from build123d import *

# Parameters (mm, degrees)
F0_R      = 5.1
F1_DEPTH  = 35
F3_START  = -5
F2_W      = 22
F2_H      = 9.65
F3_DEPTH  = 30
F4_DEPTH  = 2.5
F5_R      = 1.9
F6_DEPTH  = 20
F5_R_2    = 2.65
F7_DEPTH  = 2
F9_DEPTH  = 35
F10_COUNT = 3
F10_ANGLE = 240


with BuildPart() as f1:
    # F0 (on Top) → F1 (new body)
    with BuildSketch(Plane.XY):
        with BuildLine():
            Line((48.3891499996, -27.9374887781), (0, 0))
            Line((0, 0), (-48.3891499996, -27.9374887781))
            ThreePointArc((-48.3891499996, -27.9374887781), (-37.0005953155, -59.5433683199), (-37.3249107961, -93.1369036932))
            ThreePointArc((-37.3249107961, -93.1369036932), (-26.5643472762, -85.0438685233), (-17.5, -95))
            ThreePointArc((-17.5, -95), (-20.4289321881, -102.0710678119), (-27.5, -105))
            Line((-27.5, -105), (27.5, -105))
            ThreePointArc((27.5, -105), (19.7983455327, -88.6215583043), (37.3249107961, -93.1369036932))
            ThreePointArc((37.3249107961, -93.1369036932), (37.0005953155, -59.5433683199), (48.3891499996, -27.9374887781))
        make_face()
        with BuildLine():
            ThreePointArc((-17.5, -95), (-26.5643472762, -85.0438685233), (-37.3249107961, -93.1369036932))
            ThreePointArc((-37.3249107961, -93.1369036932), (-35.2016544673, -101.3784416957), (-27.5, -105))
            ThreePointArc((-27.5, -105), (-20.4289321881, -102.0710678119), (-17.5, -95))
        make_face()
        with Locations((-27.5, -95)):
            Circle(F0_R, mode=Mode.SUBTRACT)
        with BuildLine():
            ThreePointArc((37.5, -95), (37.4561314767, -94.0643472762), (37.3249107961, -93.1369036932))
            ThreePointArc((37.3249107961, -93.1369036932), (19.7983455327, -88.6215583043), (27.5, -105))
            ThreePointArc((27.5, -105), (34.5710678119, -102.0710678119), (37.5, -95))
        make_face()
        with Locations((27.5, -95)):
            Circle(F0_R, mode=Mode.SUBTRACT)
    extrude(amount=-F1_DEPTH)

    # F2 (on face) → F3 (cut)
    with BuildSketch(Plane.XY.offset(F3_START)):
        with Locations((0, -95.005)):
            Rectangle(F2_W, F2_H)
    extrude(amount=-F3_DEPTH, mode=Mode.SUBTRACT)

    # F0 (on Top) → F4 (join)
    with BuildSketch(Plane.XY):
        with Locations((-27.5, -95)):
            Circle(F0_R)
        with Locations((27.5, -95)):
            Circle(F0_R)
    extrude(amount=-F4_DEPTH)

    # F5 (on face) → F6 (cut)
    with BuildSketch(Plane.XZ.offset(105)):
        with Locations((0, -20)):
            Circle(F5_R)
    extrude(amount=-F6_DEPTH, mode=Mode.SUBTRACT)

    # F5 (on face) → F7 (cut)
    with BuildSketch(Plane.XZ.offset(105)):
        with Locations((0, -20)):
            Circle(F5_R_2)
        with Locations((0, -20)):
            Circle(F5_R, mode=Mode.SUBTRACT)
    extrude(amount=-F7_DEPTH, mode=Mode.SUBTRACT)

    # F8 (on face) → F9 (cut, through all)
    with BuildSketch(Plane(origin=(0, 0, -35), x_dir=(1, 0, 0), z_dir=(0, 0, -1))):
        Polygon((20.1000036855, 95.005), (20.1000036855, 99.83), (13.2999987654, 99.83), (13.2999987654, 95.005), (13.2999987654, 79.43), (20.1000036855, 79.43), align=None)
    extrude(amount=-F9_DEPTH, mode=Mode.SUBTRACT)

    # F10: F1 ×3 about axis
    f10_axis = Axis((0, 0, 0), (0, 0, 1))


with BuildPart() as f1_1:
    add(f1.part)
    for i in range(1, F10_COUNT):
        add(f1.part.rotate(f10_axis, i * F10_ANGLE / (F10_COUNT - 1)))


solid = f1_1.part
Can you work these out from the model? Positions are in its coordinate system, mm. A direction names the side the tool comes from. Round coordinates to 2 decimals unless told otherwise and drop trailing zeros. Loops run counter-clockwise (first coordinate to the right, second up) from the corner with the lowest first, then second, coordinate; pieces in that order, holes last. Notation, with made-up numbers: (-19.75, 67) - (-13.75, 67) arc R21 ccw to (-13.75, 72) - close; hole circle Ø5 at (13, 86.25). An arc over 180 degrees is marked (long way). Answer in a Markdown table with one row per item. Add a question column.
Q1. I want a section at A-A on z = -12.5. Count the separate pieces of the cut face and the enclosed holes in it, and give its area (3 significant figures).
Q2. Which directions (+Z, -Z, +X, -X, +Y, -Y) give clear straight access to the entire face, cutting with the end or side of a thin tool? Please do faces 1 (the flat face through (27, -95, -2.5)), 2 (the flat face through (-87.548, 27.336, -17.745)), 3 (the flat face through (10, -4, -35)).
Q3. For pin 1 Ø5 at (y, z) = (-93.5, -14) entering from -X; pin 2 Ø3 at (y, z) = (47.5, -28.5) entering from -X; pin 3 Ø17.5 at (x, z) = (-0.5, -15.5) entering from +Y, each with a flat end and sliding along its axis, tell me the tip position at first contact or that it passes through.
Q4. I want a section at B-B on y = -20.5. List the corners of the cut face in (x, z) for me.
Q5. We'd pull the mould along X, two halves only. Please class faces 4 (the flat face through (-90.74, 52.83, -13.37)), 5 (the flat face through (91.125, 52.167, -13.366)), 6 (the flat face through (0, -95, -5)): pulls with the +X half, pulls with the -X half, needs draft (parallel to the pull), parting line crosses it, or undercut.
Q6. I want a section at C-C on y = -74. List the corners of the cut face in (x, z) for me, and give its area (3 significant figures).
Q7. I need wall thicknesses on L1, parallel to Y at x = -87.5, z = -28; L2, parallel to Z at x = 0, y = -100; L3, parallel to Y at x = 77, z = -13. Which ranges of each line are inside material? Lowest first, please.
A:
| question | item | result |
|---|---|---|
| 1 | separate pieces | 1 |
| 1 | enclosed holes | 12 |
| 1 | area | 20,200 mm^2 |
| 2 | face 1 | -Z |
| 2 | face 2 | +Z, -Z |
| 2 | face 3 | -Z, +X, -X, +Y, -Y |
| 3 | pin 1 | x = -37.5 |
| 3 | pin 2 | x = -94.69 |
| 3 | pin 3 | y = 56.33 |
| 4 | outline | (-53.16, -35) - (53.16, -35) - (53.16, 0) - (-53.16, 0) - close |
| 5 | face 4 | pulls with the -X half |
| 5 | face 5 | pulls with the +X half |
| 5 | face 6 | undercut |
| 6 | outline | (-35.67, -35) - (35.67, -35) - (35.67, 0) - (-35.67, 0) - close |
| 6 | area | 2,500 mm^2 |
| 7 | L1 | 9.19 to 27.31, 35.16 to 37.82, 48.11 to 58.45 |
| 7 | L2 | -35 to -21.9, -18.1 to 0 |
| 7 | L3 | 2.96 to 46.99, 57.16 to 59.81, 66.29 to 76.62 |
